from build123d import *

# Parameters (mm, degrees)
F0_W     = 15
F0_H     = 3.175
F0_W_2   = 7.5
F1_DEPTH = 3.175


# Not quite as in the source:
# - a feature names something its author has since deleted; it is built from what else it names


with BuildPart() as f1:
    # F0 (on Front) → F1 (new body)
    with BuildSketch(Plane.XZ):
        Polygon((0, 28.5), (-28.5, 28.5), (-28.5, -28.5), (-13.5, -28.5), (-7.5, -28.5), (0, -28.5), (7.5, -28.5), (13.5, -28.5), (28.5, -28.5), (28.5, 23.5), (28.5, 28.5), (23.5, 28.5), align=None)
        with BuildLine():
            Line((-20.95, 23.5), (0, 23.5))
            Line((0, 23.5), (20.95, 23.5))
            ThreePointArc((20.95, 23.5), (23.5, 26.05), (26.05, 23.5))
            ThreePointArc((26.05, 23.5), (25.303122292, 21.696877708), (23.5, 20.95))
            Line((23.5, 20.95), (23.5, -20.95))
            ThreePointArc((23.5, -20.95), (25.303122292, -21.696877708), (26.05, -23.5))
            ThreePointArc((26.05, -23.5), (23.5, -26.05), (20.95, -23.5))
            Line((20.95, -23.5), (-20.95, -23.5))
            ThreePointArc((-20.95, -23.5), (-25.303122292, -25.303122292), (-23.5, -20.95))
            Line((-23.5, -20.95), (-23.5, 20.95))
            ThreePointArc((-23.5, 20.95), (-25.303122292, 25.303122292), (-20.95, 23.5))
        make_face(mode=Mode.SUBTRACT)
        with BuildLine():
            Line((-28.5, -28.5), (-28.5, 28.5))
            Line((-28.5, 28.5), (-28.5, 44))
            Line((-28.5, 44), (-51.25, 44))
            ThreePointArc((-51.25, 44), (-53.8128156646, 37.8128156646), (-60, 35.25))
            Line((-60, 35.25), (-60, -28.5))
            Line((-60, -28.5), (-49.5, -28.5))
            Line((-49.5, -28.5), (-34.5, -28.5))
            Line((-34.5, -28.5), (-28.5, -28.5))
        make_face()
        with BuildLine():
            Line((20.95, 23.5), (0, 23.5))
            Line((0, 23.5), (-20.95, 23.5))
            ThreePointArc((-20.95, 23.5), (-21.696877708, 21.696877708), (-23.5, 20.95))
            Line((-23.5, 20.95), (-23.5, -20.95))
            ThreePointArc((-23.5, -20.95), (-21.696877708, -21.696877708), (-20.95, -23.5))
            Line((-20.95, -23.5), (20.95, -23.5))
            ThreePointArc((20.95, -23.5), (21.696877708, -21.696877708), (23.5, -20.95))
            Line((23.5, -20.95), (23.5, 20.95))
            ThreePointArc((23.5, 20.95), (21.696877708, 21.696877708), (20.95, 23.5))
        make_face()
        with BuildLine():
            ThreePointArc((19.05, 0), (-13.4703841816, -13.4703841816), (0, 19.05))
            ThreePointArc((0, 19.05), (13.4703841816, 13.4703841816), (19.05, 0))
        make_face(mode=Mode.SUBTRACT)
        with BuildLine():
            Line((-51.25, 44), (-28.5, 44))
            Line((-28.5, 44), (-28.5, 60.5991594493))
            Line((-28.5, 60.5991594493), (-73.5, 60.5991594493))
            ThreePointArc((-73.5, 60.5991594493), (-77.0355339059, 59.1346933553), (-78.5, 55.5991594493))
            Line((-78.5, 55.5991594493), (-78.5, -11.5))
            ThreePointArc((-78.5, -11.5), (-73.1911039749, -24.2888484433), (-60, -28.5))
            Line((-60, -28.5), (-60, 35.25))
            ThreePointArc((-60, 35.25), (-66.1871843354, 50.1871843354), (-51.25, 44))
        make_face()
        with BuildLine():
            Line((0, 40.9), (0, 28.5))
            Line((0, 28.5), (23.5, 28.5))
            Line((23.5, 28.5), (28.5, 28.5))
            Line((28.5, 28.5), (28.5, 55.5991594493))
            ThreePointArc((28.5, 55.5991594493), (27.0355339059, 59.1346933553), (23.5, 60.5991594493))
            Line((23.5, 60.5991594493), (-28.5, 60.5991594493))
            Line((-28.5, 60.5991594493), (-28.5, 44))
            Line((-28.5, 44), (-3.1, 44))
            ThreePointArc((-3.1, 44), (0, 47.1), (3.1, 44))
            ThreePointArc((3.1, 44), (2.1920310217, 41.8079689783), (0, 40.9))
        make_face()
        with BuildLine():
            Line((-28.5, 44), (-28.5, 28.5))
            Line((-28.5, 28.5), (0, 28.5))
            Line((0, 28.5), (0, 40.9))
            ThreePointArc((0, 40.9), (-2.1920310217, 41.8079689783), (-3.1, 44))
            Line((-3.1, 44), (-28.5, 44))
        make_face()
        with Locations((21, -30.0875)):
            Rectangle(F0_W, F0_H)
        with Locations((-21, -30.0875)):
            Rectangle(F0_W, F0_H)
        with Locations((-42, -30.0875)):
            Rectangle(F0_W, F0_H)
        with Locations((3.75, -30.0875)):
            Rectangle(F0_W_2, F0_H)
        with Locations((-3.75, -30.0875)):
            Rectangle(F0_W_2, F0_H)
    extrude(amount=F1_DEPTH)


solid = f1.part
Check sheet for the modelled part. Datum: model origin and axes. Units: mm. A direction names the side the tool comes from. Round coordinates to 2 decimals unless told otherwise and drop trailing zeros. Write each loop counter-clockwise with the first axis right and the second up, starting at its lowest first coordinate (ties: lowest second). Pieces come first, ordered by that corner, then holes. Notation, with made-up numbers: (-8.5, -12) -> (42.5, -12) arc R36 ccw to (42.5, 25) -> close; hole circle Ø7 at (22.5, 79.25). An arc over 180 degrees is marked (long way). Answer as CSV lines item,"result". Start each with the question number.
1) Release check for a two-part mould opening along X. For faces 3 (the flat face through (-21, -2, -31.675)), 4 (the flat face through (28.5, -2, 11)), 5 (the flat face through (13.5, -2, -30)), 6 (the cylindrical face through (-77, -1.57, 59.17)) record: pulls with the +X half, pulls with the -X half, needs draft (parallel to the pull), parting line crosses it, or undercut.
2) Section check B-B on y = -2.4. Enter the section's corners in (x, z) (3 decimals).
3) Material ranges on line 1 (X direction, y = -1.3, z = 23.5); line 2 (Z direction, x = -23.5, y = -1.8) (3 decimals); line 3 (Z direction, x = -60, y = -2.2), recorded low to high. Write a range as from..to.
4) Tool access check on faces 1 (the flat face through (-24, -2, 60.599)), 2 (the flat face through (-11, -2, -28.5)). Record the directions out of +Z, -Z, +X, -X, +Y, -Y that give a thin tool (end or side, any length) a straight path to the whole face; none if there is none.
5) Section check A-A on z = 0. Enter the section's corners in (x, y) (3 decimals).
6) Go/stop test with flat-tipped pins: P1, Ø1.6, axis at x = 10, y = -2, coming from the -Z side; P2, Ø1, axis at y = -2, z = -29.5, coming from the -X side; P3, Ø1, axis at y = -1, z = 29, coming from the -X side. Record where each tip stops, or that it passes through.
Found:
1,face 3,"needs draft"
1,face 4,"pulls with the +X half"
1,face 5,"undercut"
1,face 6,"pulls with the -X half"
2,outline,"(-78.5, -11.5) arc R16.459 ccw to (-60, -28.5) -> (-49.5, -28.5) -> (-49.5, -31.675) -> (-34.5, -31.675) -> (-34.5, -28.5) -> (-28.5, -28.5) -> (-28.5, -31.675) -> (-13.5, -31.675) -> (-13.5, -28.5) -> (-7.5, -28.5) -> (-7.5, -31.675) -> (7.5, -31.675) -> (7.5, -28.5) -> (13.5, -28.5) -> (13.5, -31.675) -> (28.5, -31.675) -> (28.5, 55.599) arc R5 ccw to (23.5, 60.599) -> (-73.5, 60.599) arc R5 ccw to (-78.5, 55.599) -> close; hole circle Ø17.5 at (-60, 44); hole circle Ø5.1 at (-23.5, -23.5); hole circle Ø5.1 at (-23.5, 23.5); hole circle Ø38.1 at (0, 0); hole circle Ø6.2 at (0, 44); hole circle Ø5.1 at (23.5, -23.5); hole circle Ø5.1 at (23.5, 23.5)"
3,line 1,"x = -78.5..-26.05, -20.95..20.95, 26.05..28.5"
3,line 2,"z = -31.675..-26.05, -20.95..20.95, 26.05..60.599"
3,line 3,"z = -28.5..35.25, 52.75..60.6"
4,face 1,"+Z, +X, -X, +Y, -Y"
4,face 2,"-Z, +Y, -Y"
5,outline,"(-78.5, -3.175) -> (-19.05, -3.175) -> (-19.05, 0) -> (-78.5, 0) -> close; (19.05, -3.175) -> (28.5, -3.175) -> (28.5, 0) -> (19.05, 0) -> close"
6,P1,"stops at z = -28.5"
6,P2,"stops at x = -49.5"
6,P3,"stops at x = -78.5"
